from build123d import *

# Parameters (mm, degrees)
BOSS_EXTRUDE1_DEPTH = 12.7
SKETCH2_R           = 3.3782
CUT_EXTRUDE1_DEPTH  = 1.5875
FILLET2_R           = 6.35


with BuildPart() as part:
    # Sketch1 → Boss-Extrude1 (new body, symmetric)
    with BuildSketch(Plane(origin=(0, 0, 0), x_dir=(0, 0, -1), z_dir=(1, 0, 0))):
        with BuildLine():
            Line((0, 0), (0, 25.4))
            Line((0, 25.4), (6.35, 25.4))
            Line((6.35, 25.4), (6.35, 15.875))
            Line((6.35, 15.875), (25.4, 15.875))
            ThreePointArc((25.4, 15.875), (54.249114928, -62.413057838), (127, -103.2615603))
            Line((127, -103.2615603), (127, -109.848585695))
            ThreePointArc((127, -109.848585695), (51.735823624, -69.413678232), (19.05, 9.525))
            Line((19.05, 9.525), (6.35, 9.525))
            Line((6.35, 9.525), (6.35, 0))
            Line((6.35, 0), (0, 0))
        make_face()
    extrude(amount=BOSS_EXTRUDE1_DEPTH, both=True)

    # Sketch2 → Cut-Extrude1 (cut)
    with BuildSketch(Plane.XY):
        with Locations((0, 12.7)):
            Circle(SKETCH2_R)
    extrude(amount=-CUT_EXTRUDE1_DEPTH, mode=Mode.SUBTRACT)

    # Fillet2
    fillet2_edges = [part.edges().sort_by_distance(p)[0] for p in [
        (-12.7, 25.4, -3.175),
        (-12.7, 0, -3.175),
        (12.7, 25.4, -3.175),
        (12.7, 0, -3.175),
    ]]
    fillet(fillet2_edges, radius=FILLET2_R)


solid = part.part
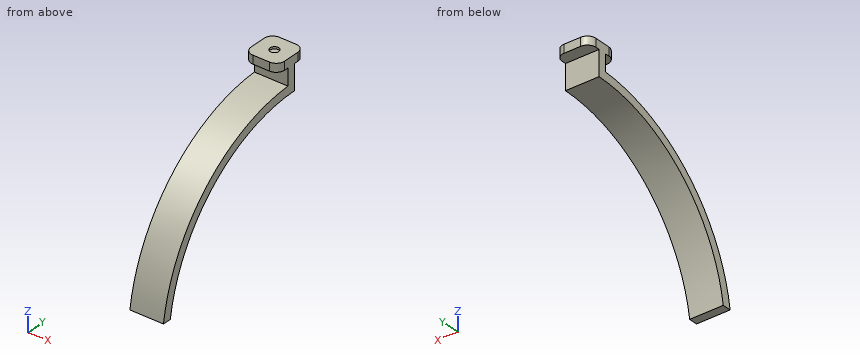
Could you check a few things on this model? Use its own coordinates, in mm. Round coordinates to 2 decimals unless told otherwise and drop trailing zeros. Write each loop counter-clockwise with the first axis right and the second up, starting at its lowest first coordinate (ties: lowest second). Pieces come first, ordered by that corner, then holes. Notation, with made-up numbers: (86.25, 38.5) -> (97.25, 38.5) arc R20 cw to (97.25, 67.5) -> close; hole circle Ø3 at (59, 38.25). An arc over 180 degrees is marked (long way). Use a Markdown table: item, result.
1. Please list where these lines run through material, in increasing order: probe 1 along Y at (x, z) = (0, -0.3); probe 2 along Z at (x, y) = (-3.5, 2); probe 3 along Y at (x, z) = (9, -15) (3 decimals).
Answer key:
| item | result |
|---|---|
| probe 1 | y = 0 to 9.32, 16.08 to 25.4 |
| probe 2 | z = -26.2 to -19.65, -6.35 to 0 |
| probe 3 | y = 9.525 to 15.875 |
2. If we section it at C-C (z = -113): List the corners of the cut face in (x, y) for me.
Answer key:
| item | result |
|---|---|
| outline | (-12.7, -106.91) -> (12.7, -106.91) -> (12.7, -100.16) -> (-12.7, -100.16) -> close |
3. If we section it at B-B (y = 12.7): List the corners of the cut face in (x, z) for me, then the cut area to 3 significant figures.
Answer key:
| item | result |
|---|---|
| outline | (-12.7, -25.44) -> (12.7, -25.44) -> (12.7, 0) -> (3.38, 0) -> (3.38, -1.59) -> (-3.38, -1.59) -> (-3.38, 0) -> (-12.7, 0) -> close |
| area | 635 mm^2 |
4. If we section it at D-D (x = 9.5): List the corners of the cut face in (y, z) for me (3 decimals).
Answer key:
| item | result |
|---|---|
| outline | (-109.849, -127) -> (-103.262, -127) arc R120.65 cw to (15.875, -25.4) -> (15.875, -6.35) -> (24.564, -6.35) -> (24.564, 0) -> (0.836, 0) -> (0.836, -6.35) -> (9.525, -6.35) -> (9.525, -19.05) arc R127.159 ccw to start |
5. For pin 1 Ø5 at (x, y) = (0.5, 4.5) entering from -Z; pin 2 Ø12 at (x, z) = (-9, -98) entering from -Y; pin 3 Ø1 at (x, z) = (7.5, -64) entering from +Y, each with a flat end and sliding along its axis, tell me the tip position at first contact or that it passes through.
Answer key:
| item | result |
|---|---|
| pin 1 | stops at z = -26.2 |
| pin 2 | stops at y = -104.13 |
| pin 3 | stops at y = -72.11 |
